Build history of the part. All positions in model axes, mm. Round coordinates to 2 decimals unless told otherwise and drop trailing zeros. Write each loop counter-clockwise with the first axis right and the second up, starting at its lowest first coordinate (ties: lowest second). Pieces come first, ordered by that corner, then holes.
from build123d import *

# Parameters (mm, degrees)
F0_W     = 110.8541414142
F0_H     = 71.3585466146
F2_DEPTH = 25.4
F1_R     = 22.5809105665


with BuildPart() as f2:
    # F0 (on Top) → F2 (new body)
    with BuildSketch(Plane.XY):
        with Locations((7.4085779488, 1.4397576451)):
            Rectangle(F0_W, F0_H)
    extrude(amount=F2_DEPTH)


with BuildPart() as f2b:
    # F1 (on Top) → F2, piece 2 (new body)
    with BuildSketch(Plane.XY):
        with Locations((33.6664095521, 0)):
            Circle(F1_R)
    extrude(amount=F2_DEPTH)


with BuildPart() as f2_1:
    add(f2.part)

    # F3: cut F2b
    add(f2b.part, mode=Mode.SUBTRACT)


solid = f2_1.part
1) Wall check: L1, parallel to Y at x = 27, z = 17.25; L2, parallel to X at y = -3, z = 12; L3, parallel to Y at x = 32, z = 8.5. Give the ranges that are in metal, low to high.
Results:
L1: y = -34.24 to -21.57, 21.57 to 37.12
L2: x = -48.02 to 11.29, 56.05 to 62.84
L3: y = -34.24 to -22.52, 22.52 to 37.12
2) Slice it at B-B (x = 15.5). Write the cut outline in (y, z).
Results:
outline: (-34.24, 0) - (-13.41, 0) - (-13.41, 25.4) - (-34.24, 25.4) - close; (13.41, 0) - (37.12, 0) - (37.12, 25.4) - (13.41, 25.4) - close
3) Slice it at A-A (y = 0). Write the cut outline in (x, z), plus the area to 3 significant figures.
Results:
outline: (-48.02, 0) - (11.09, 0) - (11.09, 25.4) - (-48.02, 25.4) - close; (56.25, 0) - (62.84, 0) - (62.84, 25.4) - (56.25, 25.4) - close
area: 1,670 mm2
4) Mould opens along Y. For faces 1 (the cylindrical face through (54.525, -8.649, 12.522)), 2 (the flat face through (7, 37.119, 13)), 3 (the flat face through (7, -34.24, 13)), 4 (the flat face through (-6, 2, 0)) say: released by +Y, released by -Y, zero draft, split by the parting line, or undercut.
Results:
face 1: undercut
face 2: released by +Y
face 3: released by -Y
face 4: zero draft
5) Pin check, flat tip, straight feed: pin 1 Ø2 at (x, y) = (-29.5, -5.5) entering from -Z. Stop position of the tip, or through.
Results:
pin 1: stops at z = 0
6) Slice it at C-C (z = 6.25). Write the cut outline in (x, y).
Results:
outline: (-48.02, -34.24) - (62.84, -34.24) - (62.84, 37.12) - (-48.02, 37.12) - close; hole circle Ø45.16 at (33.67, 0)
